Verification items for this drawing (mm, ordinates from the low corner). A direction names the side the tool comes from. Round coordinates to 2 decimals unless told otherwise and drop trailing zeros. Order: outer loops, then holes, each group sorted by start corner. A loop starts at its lowest first (then second) coordinate and runs counter-clockwise, first axis right, second up. Notation, with made-up numbers: (67, 85.5) -> (72, 85.5) arc R17 ccw to (72, 111.5) -> close; hole circle Ø5 at (47.25, 9.5). An arc over 180 degrees is marked (long way). Answer in a Markdown table with one row per item.
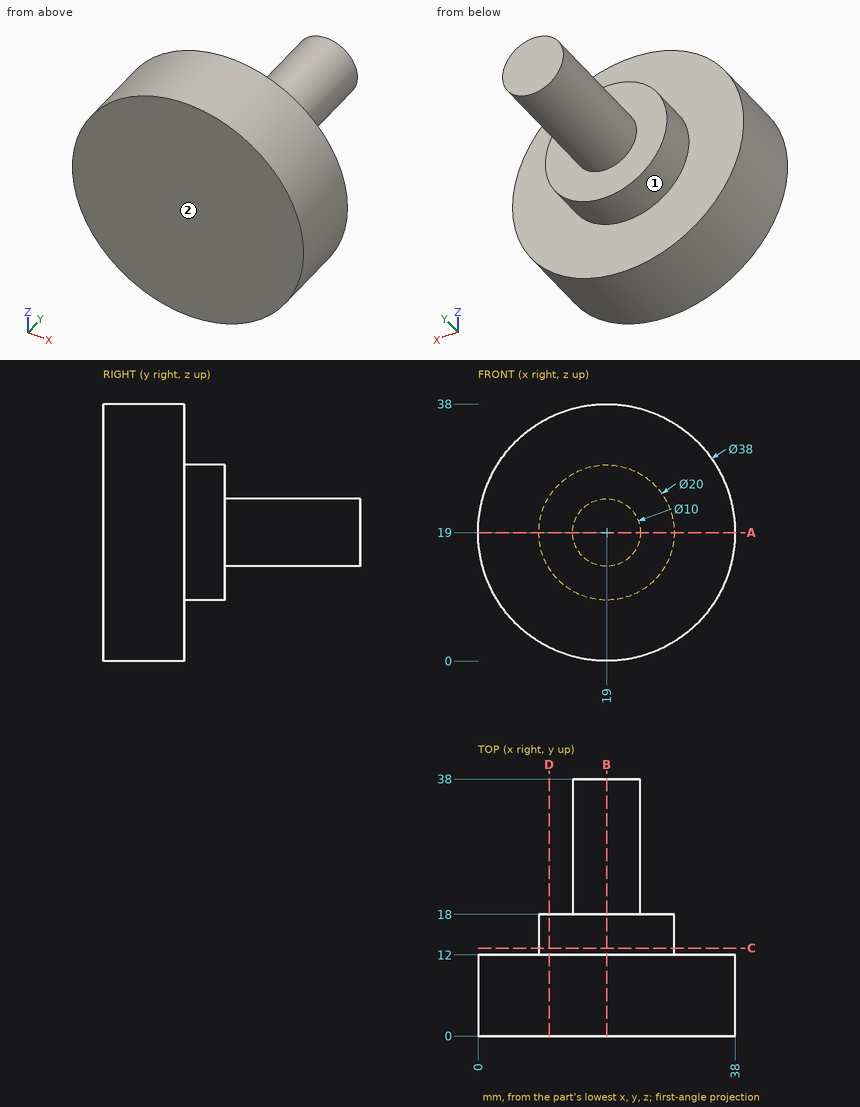
Item 1: Set-up check for the marked faces 1 and 2: record each of +Z, -Z, +X, -X, +Y, -Y from which the full face is reachable in a straight line by a thin tool's end or side.
Result sheet:
| item | result |
|---|---|
| face 1 | +Y |
| face 2 | +Z, -Z, +X, -X, -Y |
Item 2: Cross-section at D-D (x = 10.5). Record the boundary of the cut face in (y, z).
Result sheet:
| item | result |
|---|---|
| outline | (0, 2.01) -> (12, 2.01) -> (12, 13.73) -> (18, 13.73) -> (18, 24.27) -> (12, 24.27) -> (12, 35.99) -> (0, 35.99) -> close |
Item 3: Depth check by flat-ended pin: P1, Ø5, axis at x = 6, z = 23, coming from the -Y side; P2, Ø1, axis at x = 23.5, y = 6.5, coming from the +Z side; P3, Ø10, axis at x = 26, z = 5.5, coming from the +Y side; P4, Ø3, axis at x = 34, y = 4, coming from the -Z side. Enter the tip coordinate at first touch or a pass-through.
Result sheet:
| item | result |
|---|---|
| P1 | stops at y = 0 |
| P2 | stops at z = 37.57 |
| P3 | stops at y = 12 |
| P4 | stops at z = 5.63 |
Item 4: Cross-section at B-B (x = 19). Record the boundary of the cut face in (y, z).
Result sheet:
| item | result |
|---|---|
| outline | (0, 0) -> (12, 0) -> (12, 9) -> (18, 9) -> (18, 14) -> (38, 14) -> (38, 24) -> (18, 24) -> (18, 29) -> (12, 29) -> (12, 38) -> (0, 38) -> close |
Item 5: Scan lines: line 1 (Y direction, x = 20, z = 29); line 2 (Z direction, x = 19, y = 3.5); line 3 (Y direction, x = 28, z = 22). Record each from-to range of solid material in increasing order. Write a range as [from, to].
Result sheet:
| item | result |
|---|---|
| line 1 | y = [0, 12] |
| line 2 | z = [0, 38] |
| line 3 | y = [0, 18] |
Item 6: Cross-section at C-C (y = 13). Record the boundary of the cut face in (x, z).
Result sheet:
| item | result |
|---|---|
| outline | circle Ø20 at (19, 19) |
Item 7: Cross-section at A-A (z = 19). Record the boundary of the cut face in (x, y), and give its area (3 significant figures).
Result sheet:
| item | result |
|---|---|
| outline | (0, 0) -> (38, 0) -> (38, 12) -> (29, 12) -> (29, 18) -> (24, 18) -> (24, 38) -> (14, 38) -> (14, 18) -> (9, 18) -> (9, 12) -> (0, 12) -> close |
| area | 776 mm^2 |
